from build123d import *

# Parameters (mm, degrees)
F1_DEPTH = 100
F3_DEPTH = 5


with BuildPart() as f1:
    # F0 (on Top) → F1 (new body)
    with BuildSketch(Plane.XY):
        with BuildLine():
            Line((-20, 0), (20, 0))
            ThreePointArc((20, 0), (0, 20), (-20, 0))
        make_face()
        with BuildLine():
            Line((20, -25), (20, 0))
            ThreePointArc((20, 0), (0, -20), (-20, 0))
            Line((-20, 0), (-20, -25))
            Line((-20, -25), (20, -25))
        make_face()
        with BuildLine():
            ThreePointArc((-20, 0), (0, -20), (20, 0))
            Line((20, 0), (-20, 0))
        make_face()
    extrude(amount=F1_DEPTH)

    # F2 (on face) → F3 (join)
    with BuildSketch(Plane.XY.offset(100)):
        with BuildLine():
            Line((-20, 10), (-20, 0))
            Line((-20, 0), (30, 0))
            Line((30, 0), (30, 10))
            ThreePointArc((30, 10), (5, 35), (-20, 10))
        make_face()
    extrude(amount=F3_DEPTH)


solid = f1.part
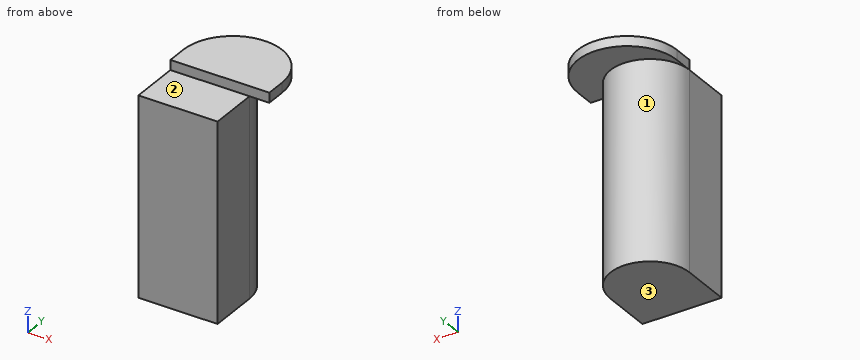
Design review of the part built by this model. Coordinates are the model's own, in mm. Face numbers are marked on the shaded views. A direction names the side the tool comes from. Give positions to 0.01 mm unless a question says otherwise; leave off trailing zeros. Loops run counter-clockwise (first coordinate to the right, second up) from the corner with the lowest first, then second, coordinate; pieces in that order, holes last. Notation, with made-up numbers: (18.25, 59.5) - (33.25, 59.5) arc R17 cw to (33.25, 92.5) - close; hole circle Ø5 at (46.5, 79). An arc over 180 degrees is marked (long way). Use CSV: the item, a comma, the result in double quotes. Start each with the question number.
1. Add section C-C (z = 63.5). State the section outline as (x, y) points.
2. Machinability: for the marked faces 1, 2 and 3, which of the approach directions +Z, -Z, +X, -X, +Y, -Y give a long, thin tool a straight path to every point of the face, cutting with its end or side? Answer none if there is none.
3. Insertion check: P1, Ø6, axis at x = 4, z = 82.5, coming from the +Y side (3 decimals); P2, Ø7.5, axis at x = 5.5, y = -9, coming from the +Z side; P3, Ø1.5, axis at x = 7.5, y = 22.5, coming from the -Z side. Each pin has a flat end and moves straight along its axis. Give the tip position at first contact, or say it passes through.
4. Add section B-B (x = 5). State the section outline as (y, z) points.
5. Add section A-A (y = 1.5). State the section outline as (x, z) points.
6. Wall thickness on L1, parallel to Y at x = 0, z = 6; L2, parallel to X at y = -7, z = 58.5; L3, parallel to Z at x = -15, y = 17.5: over which ranges is each line inside the solid? List them lowest first.
Results found:
1,outline,"(-20, -25) - (20, -25) - (20, 0) arc R20 ccw to (-20, 0) - close"
2,face 1,"-Z, +Y"
2,face 2,"+Z, +X, -X, -Y"
2,face 3,"-Z, +X, -X, +Y, -Y"
3,P1,"stops at y = 19.975"
3,P2,"stops at z = 100"
3,P3,"stops at z = 100"
4,outline,"(-25, 0) - (19.36, 0) - (19.36, 100) - (35, 100) - (35, 105) - (0, 105) - (0, 100) - (-25, 100) - close"
5,outline,"(-20, 100) - (-19.94, 100) - (-19.94, 0) - (19.94, 0) - (19.94, 100) - (30, 100) - (30, 105) - (-20, 105) - close"
6,L1,"y = -25 to 20"
6,L2,"x = -20 to 20"
6,L3,"z = 100 to 105"
